```python
from build123d import *

# Parameters (mm, degrees)
F0_R      = 75
F1_DEPTH  = 5
F0_R_2    = 79
F2_DEPTH  = 30
F3_R      = 142.5
F3_R_2    = 79
F3_R_3    = 75
F4_DEPTH  = 5
F3_R_4    = 145.5
F5_DEPTH  = 158
F6_DEPTH  = 180
F7_R      = 150.5
F7_R_2    = 145.5
F7_R_3    = 142.5
F8_DEPTH  = 7.5
F9_R      = 150.5
F9_R_2    = 147
F10_DEPTH = 13
F11_R     = 6.5
F11_R_2   = 3.5
F12_DEPTH = 7
F13_D     = 6.6
F13_DEPTH = 12
F13_TIP   = 1.9828400428


with BuildPart() as f1:
    # F0 (on Top) → F1 (new body)
    with BuildSketch(Plane.XY):
        Circle(F0_R)
        with BuildLine():
            ThreePointArc((-27.2772727273, 3.4929060339), (0, 27.5), (27.2772727273, 3.4929060339))
            ThreePointArc((27.2772727273, 3.4929060339), (31, 0), (27.2772727273, -3.4929060339))
            ThreePointArc((27.2772727273, -3.4929060339), (0, -27.5), (-27.2772727273, -3.4929060339))
            ThreePointArc((-27.2772727273, -3.4929060339), (-31, 0), (-27.2772727273, 3.4929060339))
        make_face(mode=Mode.SUBTRACT)
    extrude(amount=F1_DEPTH)

    # F0 (on Top) → F2 (join)
    with BuildSketch(Plane.XY):
        Circle(F0_R_2)
        Circle(F0_R, mode=Mode.SUBTRACT)
    extrude(amount=F2_DEPTH)

    # F3 (on face) → F4 (join)
    with BuildSketch(Plane.XY.offset(30)):
        Circle(F3_R)
        Circle(F3_R_2, mode=Mode.SUBTRACT)
        Circle(F3_R_2)
        Circle(F3_R_3, mode=Mode.SUBTRACT)
    extrude(amount=F4_DEPTH)

    # F3 (on face) → F5 (join)
    with BuildSketch(Plane.XY.offset(30)):
        Circle(F3_R_4)
        Circle(F3_R, mode=Mode.SUBTRACT)
    extrude(amount=F5_DEPTH)

    # F3 (on face) → F6 (join)
    with BuildSketch(Plane.XY.offset(30)):
        Circle(F3_R_4)
        Circle(F3_R, mode=Mode.SUBTRACT)
    extrude(amount=-F6_DEPTH)

    # F7 (on face) → F8 (join)
    with BuildSketch(Plane(origin=(0, 0, -150), x_dir=(1, 0, 0), z_dir=(0, 0, -1))):
        Circle(F7_R)
        Circle(F7_R_2, mode=Mode.SUBTRACT)
        Circle(F7_R_2)
        Circle(F7_R_3, mode=Mode.SUBTRACT)
    extrude(amount=F8_DEPTH)

    # F9 (on face) → F10 (join)
    with BuildSketch(Plane(origin=(0, 0, -157.5), x_dir=(1, 0, 0), z_dir=(0, 0, -1))):
        Circle(F9_R)
        Circle(F9_R_2, mode=Mode.SUBTRACT)
    extrude(amount=F10_DEPTH)

    # F11 (on face) → F12 (join)
    with BuildSketch(Plane.XY.offset(35)):
        with Locations((0, 82.1006134727)):
            Circle(F11_R)
        with Locations((0, 82.1006134727)):
            Circle(F11_R_2, mode=Mode.SUBTRACT)
        with Locations((65.5, -49.5001084099)):
            Circle(F11_R)
        with Locations((65.5, -49.5001084099)):
            Circle(F11_R_2, mode=Mode.SUBTRACT)
        with Locations((-65.5, -49.5001084099)):
            Circle(F11_R)
        with Locations((-65.5, -49.5001084099)):
            Circle(F11_R_2, mode=Mode.SUBTRACT)
    extrude(amount=F12_DEPTH)

    # F13
    with Locations(Plane.XY.offset(35)):
        with Locations((0, 82.1006134727), (65.5, -49.5001084099), (-65.5, -49.5001084099)):
            Hole(F13_D / 2, depth=F13_DEPTH)
            with Locations((0, 0, -(F13_DEPTH + F13_TIP / 2))):  # 118° drill point
                Cone(0, F13_D / 2, F13_TIP, mode=Mode.SUBTRACT)


solid = f1.part
```
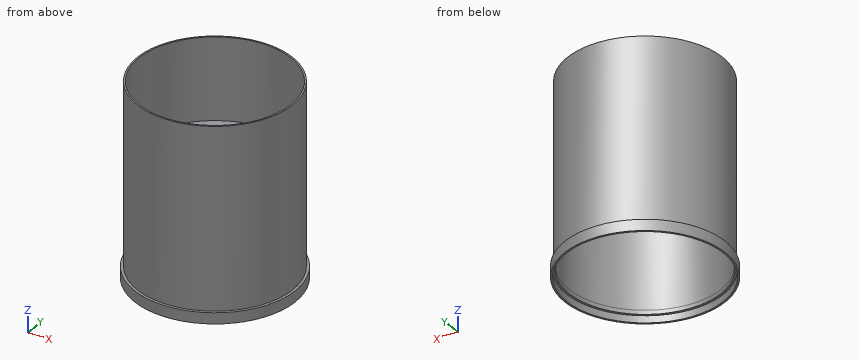
The model under review builds one solid part; all positions refer to its coordinate system, in mm. Coordinates: 2 decimals unless noted, no trailing zeros. Write each loop counter-clockwise with the first axis right and the second up, starting at its lowest first coordinate (ties: lowest second). Pieces come first, ordered by that corner, then holes.
1) We need section C-C on y = -111. State the section outline as (x, z) points.
2) We need section A-A on z = 10. State the section outline as (x, y) points.
3) Clearance check with flat-ended pins moving along their axes: pin 1 Ø7.5 at (x, y) = (65.5, -49.5) entering from +Z; pin 2 Ø4 at (x, z) = (-83, 119) entering from -Y; pin 3 Ø12 at (x, z) = (-64, 62.5) entering from +Y. State where each tip first meets the part, or that it passes through.
4) We need section D-D on z = -28. State the section outline as (x, y) points.
5) To check wall thickness, follow probe 1 along Y at (x, z) = (0, 19); probe 2 along Y at (x, z) = (0, -167); probe 3 along Y at (x, z) = (0, -152.25). State the ranges of each line that lie inside material, in increasing order.
Answer list:
1. outline: (-101.63, -170.5) - (-96.37, -170.5) - (-96.37, -157.5) - (-89.36, -157.5) - (-89.36, 30) - (89.36, 30) - (89.36, -157.5) - (96.37, -157.5) - (96.37, -170.5) - (101.63, -170.5) - (101.63, -150) - (94.07, -150) - (94.07, 188) - (89.36, 188) - (89.36, 35) - (-89.36, 35) - (-89.36, 188) - (-94.07, 188) - (-94.07, -150) - (-101.63, -150) - close
2. outline: circle Ø291 at (0, 0); circle Ø158 at (0, 0); hole circle Ø285 at (0, 0); hole circle Ø150 at (0, 0)
3. pin 1: stops at z = 42
3. pin 2: stops at y = -120.87
3. pin 3: stops at y = 133.44
4. outline: circle Ø291 at (0, 0); hole circle Ø285 at (0, 0)
5. probe 1: y = -145.5 to -142.5, -79 to -75, 75 to 79, 142.5 to 145.5
5. probe 2: y = -150.5 to -147, 147 to 150.5
5. probe 3: y = -150.5 to -142.5, 142.5 to 150.5
